Verification items for the finished model (mm, model axes). Coordinates: 2 decimals unless noted, no trailing zeros. Write each loop counter-clockwise with the first axis right and the second up, starting at its lowest first coordinate (ties: lowest second). Pieces come first, ordered by that corner, then holes. Notation, with made-up numbers: (70.5, 25.5) -> (123.5, 25.5) arc R29 cw to (123.5, 45.5) -> close; hole circle Ø7 at (41.5, 20.5). An arc over 180 degrees is marked (long way). Use CSV: the item, a comma, the result in double quotes.
Autodesk Inventor part; units mm, degrees
ref_plane "YZ Plane" through (0, 0, 0) normal (1, 0, 0) x (0, 1, 0)
ref_plane "XZ Plane" through (0, 0, 0) normal (0, 1, 0) x (-1, 0, 0)
ref_plane "XY Plane" through (0, 0, 0) normal (0, 0, 1) x (1, 0, 0)
sketch "Sketch1" plane through (0, 0, 0) normal (0, 1, 0) x (-1, 0, 0)
  line L0 (-2.5781, 12.7) -> (2.5781, 12.7)
  line L1 (2.5781, 12.7) -> (2.5781, -12.7)
  line L2 (2.5781, -12.7) -> (-2.5781, -12.7)
  line L3 (-2.5781, -12.7) -> (-2.5781, 12.7)
  line L4 (-2.5781, 12.7) -> (2.5781, -12.7) construction
  line L5 (2.5781, 12.7) -> (-2.5781, -12.7) construction
  point P0 (0, 0)
  dimension "d0" = 5.1562
  dimension "d1" = 25.4
extrude "Extrusion1" add sketch "Sketch1" along normal blind 1.1938
sketch "Sketch2" plane through (0, 1.1938, 0) normal (0, 1, 0) x (1, 0, 0)
  line L0 (2.5781, 12.7) -> (-2.5781, 12.7)
  line L1 (-2.5781, 12.7) -> (-2.5781, -12.7)
  line L2 (-2.5781, -12.7) -> (2.5781, -12.7)
  line L3 (2.5781, -12.7) -> (2.5781, 12.7)
  line L4 (-3.6093, 0) -> (3.6093, 0)
  line L5 (0, 17.78) -> (0, -17.78)
  circle A0 centre (1.27, -11.5062) radius 0.5969
  circle A1 centre (-1.27, -11.5062) radius 0.5969
  line L6 (2.5781, 12.7) -> (-2.5781, 12.7)
  line L7 (0.0508, -12.7) -> (-0.0508, -12.7)
  line L8 (-0.0508, -12.7) -> (-0.0508, 12.7)
  line L9 (-0.0508, 12.7) -> (0.0508, 12.7)
  line L10 (0.0508, 12.7) -> (0.0508, -12.7)
  line L11 (0.0508, -12.7) -> (-0.0508, 12.7) construction
  line L12 (-0.0508, -12.7) -> (0.0508, 12.7) construction
  point P0 (0, 0)
  dimension "d4" = 1.1938
  dimension "d5" = 1.1938
  dimension "d8" = 1.27
  dimension "d9" = 0.1016
extrude "Extrusion2" add sketch "Sketch2" along normal blind 0.0381 contours L3 L4 L10 L0 | L3 L2 L10 L4 | L8 L4 L1 L0 | L8 L2 L1 L4
sketch "Sketch3" plane through (1.27, 1.1938, 11.5062) normal (0, 1, 0) x (1, 0, 0)
  point P0 (-1.27, 11.5062)
sketch "Sketch4" plane through (0, 0, 0) normal (0, 1, 0) x (-1, 0, 0)
  circle A0 centre (-1.27, 11.5062) radius 0.5969
  circle A1 centre (1.27, 11.5062) radius 0.5969
  line L0 (3.6093, 0) -> (-3.6093, 0)
  line L1 (0, -17.78) -> (0, 17.78)
  line L2 (0.0508, -12.7) -> (2.5781, -12.7)
  line L3 (2.5781, -12.7) -> (2.5781, 12.7)
  line L4 (2.5781, 12.7) -> (0.0508, 12.7)
  line L5 (0.0508, 12.7) -> (0.0508, -12.7)
  circle A2 centre (1.27, 11.5062) radius 0.5969
  line L6 (-0.0508, 12.7) -> (-2.5781, 12.7)
  line L7 (-2.5781, 12.7) -> (-2.5781, -12.7)
  line L8 (-2.5781, -12.7) -> (-0.0508, -12.7)
  line L9 (-0.0508, -12.7) -> (-0.0508, 12.7)
  circle A3 centre (-1.27, 11.5062) radius 0.5969
  point P0 (0, 0)
extrude "Extrusion3" cut sketch "Sketch4" along normal through all contours A0 | A1
equation "\"BendRadius\" = Thickness"
equation "\"BendReliefWidth\" = Thickness"
equation "\"BendReliefDepth\" = 0.5 * Thickness"
equation "\"CornerReliefSize\" = 4 * Thickness"
equation "\"MinimumRemnant\" = 2 * Thickness"
equation "\"TransitionRadius\" = BendRadius"
equation "\"JacobiRadiusSize\" = BendRadius"
equation "\"GapSize\" = Thickness"
properties part number "Leads+ChannelForSingleHeater"
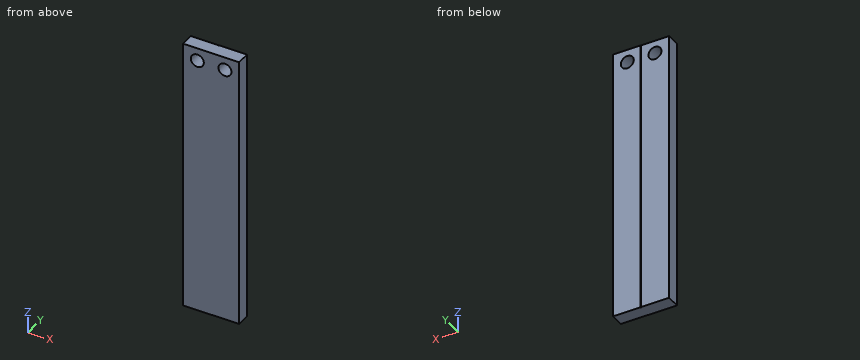
1) Gauge pin test, flat end, axial feed: pin 1 (1 mm diameter, centred on x = -1.27, z = 11.51, fed in from +Y). Record the tip position at first contact, or that the pin passes through.
Return value:
pin 1,"through"
2) Scan lines: L1, parallel to Z at x = -1.27, y = 0.8; L2, parallel to X at y = 0.1, z = 11.25; L3, parallel to Z at x = -1.05, y = 0.6. Record each from-to range of solid material in increasing order.
Return value:
L1,"-12.7 to 10.91, 12.1 to 12.7"
L2,"-2.58 to -1.81, -0.73 to 0.73, 1.81 to 2.58"
L3,"-12.7 to 10.95, 12.06 to 12.7"
3) Cross-section at A-A (x = -1.27). Record the boundary of the cut face in (y, z).
Return value:
outline,"(0, -12.7) -> (1.23, -12.7) -> (1.23, 10.91) -> (0, 10.91) -> close; (0, 12.1) -> (1.23, 12.1) -> (1.23, 12.7) -> (0, 12.7) -> close"
4) Cross-section at B-B (y = 0.35). Record the boundary of the cut face in (x, z), plus the area to 3 significant figures.
Return value:
outline,"(-2.58, -12.7) -> (2.58, -12.7) -> (2.58, 12.7) -> (-2.58, 12.7) -> close; hole circle Ø1.19 at (-1.27, 11.51); hole circle Ø1.19 at (1.27, 11.51)"
area,"129 mm2"
